Autodesk Inventor part; units mm, degrees
ref_plane "YZ Plane" through (0, 0, 0) normal (1, 0, 0) x (0, 1, 0)
ref_plane "XZ Plane" through (0, 0, 0) normal (0, 1, 0) x (-1, 0, 0)
ref_plane "XY Plane" through (0, 0, 0) normal (0, 0, 1) x (1, 0, 0)
sketch "Boceto1" plane through (0, 0, 0) normal (0, 1, 0) x (-1, 0, 0)
  circle A0 centre (0, 0) radius 4
  circle A1 centre (0, 0) radius 14
  line L0 (-7.0696, 2.75) -> (-10.0696, 2.75)
  line L1 (-10.0696, 2.75) -> (-10.0696, -2.75)
  line L2 (-10.0696, -2.75) -> (-7.0696, -2.75)
  line L3 (-7.0696, -2.75) -> (-7.0696, 2.75)
  circle A2 centre (0, 0) radius 9 construction
  point P0 (-7.0696, 0)
  point P1 (-8.5696, 2.75)
  dimension "d0" = 8
  dimension "tuerca" = 5.5
  dimension "d2" = 10
  dimension "d3" = 5
  dimension "d4" = 3
extrude "Extrusión1" add sketch "Boceto1" along normal blind 8
sketch "Boceto2" plane through (7.0696, 0, -2.75) normal (1, 0, 0) x (0, 0, -1)
  line L0 (0, 0) -> (-5.5, 0)
  line L1 (0, 0) -> (0, 8) construction
  line L2 (-5.5, 8) -> (0, 8) construction
  line L3 (-5.5, 0) -> (-5.5, 8) construction
  line L4 (-5.5, 0) -> (0, 8) construction
  circle A0 centre (-2.75, 4) radius 1.6
  line L5 (0, 2.1813) -> (-2.75, 0.5936)
  line L6 (-2.75, 0.5936) -> (-5.5, 2.1813)
  line L7 (-5.5, 2.1813) -> (-5.5, 0)
  line L8 (0, 2.1813) -> (0, 0)
  point P0 (-2.75, 0)
  dimension "d7" = 3.2
  dimension "d8" = 120
  dimension "d9" = 2.95
extrude "Extrusión2" cut sketch "Boceto2" along normal mid plane 15 contours A0
extrude "Extrusión3" add sketch "Boceto2" along normal up to next contours L0 L7 L6 L5 L8
sketch "Boceto3" plane through (0, 0, 0) normal (0, -1, 0) x (1, 0, 0)
  circle A0 centre (0, 0) radius 4
  circle A1 centre (0, 0) radius 17.939
extrude "Extrusión4" add sketch "Boceto3" along normal blind 10
equation "\"d3\" = 0.5 * d2"
properties part number "poleaT5"
CAD build for the part. Positions are in the model's coordinates, mm. A direction names the side the tool comes from. Coordinates: 2 decimals unless noted, no trailing zeros. Order: outer loops, then holes, each group sorted by start corner. A loop starts at its lowest first (then second) coordinate and runs counter-clockwise, first axis right, second up.
(1) Saw through at C-C, the plane y = -5.5. Write the cut outline in (x, z), and give its area (3 significant figures).
Solution:
outline: circle Ø35.88 at (0, 0); hole circle Ø8 at (0, 0)
area: 961 mm2
(2) Saw through at A-A, the plane x = 0. Write the cut outline in (y, z).
Solution:
outline: (-10, -17.94) - (0, -17.94) - (0, -14) - (8, -14) - (8, -4) - (-10, -4) - close; (-10, 4) - (8, 4) - (8, 14) - (0, 14) - (0, 17.94) - (-10, 17.94) - close
(3) Which spindle directions (+Z, -Z, +X, -X, +Y, -Y) get a long thin tool onto all of the face, cutting with end or side? Do faces 1 (the face through (-0.3, -10, 4.2)), 2 (the face through (9, 5, 2.75)), 3 (the face through (12.007, 2.414, 0.208)). Say none if no direction does.
Solution:
face 1: +Z, -Z, +X, -X, -Y
face 2: +Y
face 3: +X
(4) Drill centre lines: L1, parallel to X at y = 6, z = 0; L2, parallel to Z at x = 0, y = 1.25; L3, parallel to Y at x = 11.95, z = 0. Where is each one in solid material? Low to high.
Solution:
L1: x = -14 to -4, 4 to 7.07, 10.07 to 14
L2: z = -14 to -4, 4 to 14
L3: y = -10 to 2.4, 5.6 to 8
(5) Saw through at B-B, the plane x = 13. Write the cut outline in (y, z), and give its area (3 significant figures).
Solution:
outline: (-10, -12.36) - (0, -12.36) - (0, -5.2) - (8, -5.2) - (8, 5.2) - (0, 5.2) - (0, 12.36) - (-10, 12.36) - close; hole circle Ø3.2 at (4, 0)
area: 322 mm2
(6) Saw through at D-D, the plane z = 9. Write the cut outline in (x, y).
Solution:
outline: (-15.52, -10) - (15.52, -10) - (15.52, 0) - (10.72, 0) - (10.72, 8) - (-10.72, 8) - (-10.72, 0) - (-15.52, 0) - close
(7) Mould opens along X. For faces 4 (the face through (8.5, 1.4, -1.4)), 5 (the face through (5.39, 4.07, 1.6)), 6 (the face through (-3.889, -4.93, 17.512)), 7 (the face through (9, 5, -2.75)) say: released by +X, released by -X, zero draft, split by the parting line, or undercut.
Solution:
face 4: undercut
face 5: zero draft
face 6: split by the parting line
face 7: undercut
(8) Pin check, flat tips, straight feed: pin 1 Ø2.5 at (x, y) = (9, 5) entering from -Z; pin 2 Ø3 at (y, z) = (-6.5, -8) entering from +X; pin 3 Ø1 at (x, y) = (-12, -2) entering from +Z. Stop position of each tip, or through.
Solution:
pin 1: stops at z = -11.66
pin 2: stops at x = 16.72
pin 3: stops at z = 13.77
